For this review, take the finished solid that the model builds, in its own axes (mm). Face numbers are marked on the shaded views. Round coordinates to 2 decimals unless told otherwise and drop trailing zeros. Order: outer loops, then holes, each group sorted by start corner. A loop starts at its lowest first (then second) coordinate and runs counter-clockwise, first axis right, second up. Notation, with made-up numbers: (-11.5, 16) -> (31.5, 16) arc R22 ccw to (31.5, 37) -> close; hole circle Ø9 at (34.25, 79.5). An arc over 180 degrees is marked (long way). Use a Markdown table: item, result. Add a question column.
1) Consider section A-A (x = 50.8). State the section outline as (y, z) points (3 decimals).
2) Consider section C-C (x = 0). State the section outline as (y, z) points.
3) Clearance check with flat-ended pins moving along their axes: P1, Ø6, axis at x = 21, y = 19, coming from the +Z side; P2, Ø5, axis at y = 18.5, z = 18.5, coming from the +X side; P3, Ø11.5, axis at x = 50.8, z = -28.575, coming from the -Y side (3 decimals); P4, Ø12, axis at x = 15, z = -27, coming from the -Y side. State where each tip first meets the part, or that it passes through.
4) Wall thickness on line 1 along Z through (x, y) = (50.8, 7) (3 decimals); line 2 along Z through (x, y) = (0, 13); line 3 along Y through (x, z) = (30, -25): over which ranges is each line inside the solid? List them lowest first. Write a range as [from, to].
5) Consider section B-B (y = 8.5). Give the number of separate pieces and of enclosed holes in the cut face, plus the area to 3 significant figures.
6) Consider section D-D (y = 13). State the section outline as (x, z) points (1 decimal), plus the area to 3 significant figures.
7) Draft analysis for pull direction X (two halves, no side actions). For the marked faces 1, 2 and 3, state which applies: pulls with the +X half, pulls with the -X half, needs draft (parallel to the pull), parting line crosses it, or undercut.
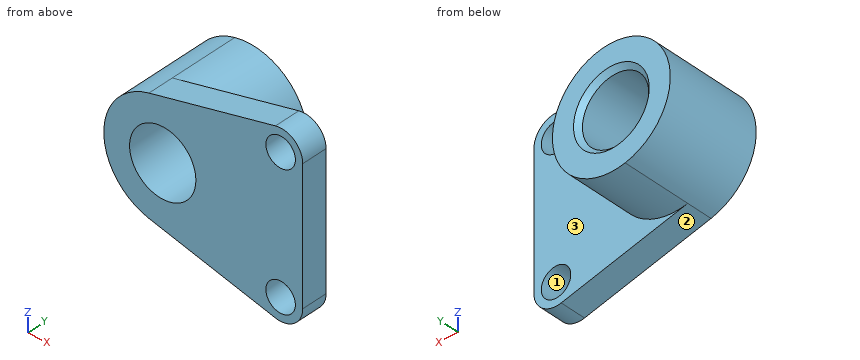
```python
from build123d import *

# Parameters (mm, degrees)
F0_R        = 14.2875
F1_DEPTH    = 41.148
F0_R_2      = 6.35
F1_FACE_R   = 25.4
F1_FACE_R_2 = 14.2875
F2_DEPTH    = 11.176
F3_SIZE2    = 2.032
F3_SIZE     = 2.032


with BuildPart() as f1:
    # F0 (on Front) → F1 (new body)
    with BuildSketch(Plane.XZ):
        with BuildLine():
            ThreePointArc((-5.9521693415, -24.692745496), (15.7158343515, -19.9542614656), (25.4, 0))
            ThreePointArc((25.4, 0), (15.7158343515, 19.9542614656), (-5.9521693415, 24.692745496))
            ThreePointArc((-5.9521693415, 24.692745496), (-25.4, 0), (-5.9521693415, -24.692745496))
        make_face()
        Circle(F0_R, mode=Mode.SUBTRACT)
    extrude(amount=-F1_DEPTH)

    # F0 (on Front) + F1_face (on face) → F2 (join)
    with BuildSketch(Plane.XZ):
        with BuildLine():
            ThreePointArc((-5.9521693415, -24.692745496), (15.7158343515, -19.9542614656), (25.4, 0))
            ThreePointArc((25.4, 0), (15.7158343515, 19.9542614656), (-5.9521693415, 24.692745496))
            ThreePointArc((-5.9521693415, 24.692745496), (-25.4, 0), (-5.9521693415, -24.692745496))
        make_face()
        Circle(F0_R, mode=Mode.SUBTRACT)
        with BuildLine():
            ThreePointArc((-5.9521693415, 24.692745496), (15.7158343515, 19.9542614656), (25.4, 0))
            ThreePointArc((25.4, 0), (15.7158343515, -19.9542614656), (-5.9521693415, -24.692745496))
            Line((-5.9521693415, -24.692745496), (48.5679364969, -37.834779561))
            ThreePointArc((48.5679364969, -37.834779561), (56.6934378818, -36.0578480496), (60.325, -28.575))
            Line((60.325, -28.575), (60.325, 28.575))
            ThreePointArc((60.325, 28.575), (56.6934378818, 36.0578480496), (48.5679364969, 37.834779561))
            Line((48.5679364969, 37.834779561), (-5.9521693415, 24.692745496))
        make_face()
        with Locations((50.8, -28.575)):
            Circle(F0_R_2, mode=Mode.SUBTRACT)
        with Locations((50.8, 28.575)):
            Circle(F0_R_2, mode=Mode.SUBTRACT)
    with BuildSketch(Plane.XZ):
        Circle(F1_FACE_R)
        Circle(F1_FACE_R_2, mode=Mode.SUBTRACT)
    extrude(amount=-F2_DEPTH)

    # F3
    f3_edges = [f1.edges().sort_by_distance(p)[0] for p in [
        (-14.2875, 41.148, 0),
    ]]
    chamfer(f3_edges, length=F3_SIZE, length2=F3_SIZE2)


solid = f1.part
```
Results list:
| question | item | result |
|---|---|---|
| 1 | outline | (0, -38.1) -> (11.176, -38.1) -> (11.176, -34.925) -> (0, -34.925) -> close; (0, -22.225) -> (11.176, -22.225) -> (11.176, 22.225) -> (0, 22.225) -> close; (0, 34.925) -> (11.176, 34.925) -> (11.176, 38.1) -> (0, 38.1) -> close |
| 2 | outline | (0, -26.13) -> (11.18, -26.13) -> (11.18, -25.4) -> (41.15, -25.4) -> (41.15, -16.32) -> (39.12, -14.29) -> (0, -14.29) -> close; (0, 14.29) -> (39.12, 14.29) -> (41.15, 16.32) -> (41.15, 25.4) -> (11.18, 25.4) -> (11.18, 26.13) -> (0, 26.13) -> close |
| 3 | P1 | z = 17.92 |
| 3 | P2 | x = 19.73 |
| 3 | P3 | through |
| 3 | P4 | y = 0 |
| 4 | line 1 | [-38.1, -34.925], [-22.225, 22.225], [34.925, 38.1] |
| 4 | line 2 | [-25.4, -14.29], [14.29, 25.4] |
| 4 | line 3 | [0, 11.18] |
| 5 | separate pieces | 1 |
| 5 | enclosed holes | 3 |
| 5 | area | 4,080 mm2 |
| 6 | outline | circle Ø50.8 at (0, 0); hole circle Ø28.6 at (0, 0) |
| 6 | area | 1,390 mm2 |
| 7 | face 1 | undercut |
| 7 | face 2 | pulls with the -X half |
| 7 | face 3 | needs draft |
